```python
from build123d import *

# Parameters (mm, degrees)
F2_W      = 42.5
F2_H      = 40.5
F2_R      = 7.5
F8_DEPTH  = 2
F6_W      = 23.5
F6_H      = 40.5
F9_DEPTH  = 2
F5_W      = 23.5
F5_H      = 40.5
F10_DEPTH = 2
F0_W      = 42.5
F0_H      = 20.5
F11_DEPTH = 2
F7_W      = 1
F7_H      = 2
F12_DEPTH = 38.5
F13_DEPTH = 40.5
F14_R     = 0.99999


# Not quite as in the source:
# - a fillet or chamfer that OpenCascade refuses, or shapes differently, is made with other operations: its cross-section is extruded or revolved along the edge and cut away or added
# - a fillet or chamfer is up to 0.001 mm smaller than in the source, because OpenCascade refuses the exact size


with BuildPart() as f8:
    # F2 (on line) → F8 (new body)
    with BuildSketch(Plane.XZ.offset(10.25)):
        with Locations((0, 20.25)):
            Rectangle(F2_W, F2_H)
        with Locations((0, 20.25)):
            Circle(F2_R, mode=Mode.SUBTRACT)
    extrude(amount=-F8_DEPTH)

    # F6 (on line) → F9 (join)
    with BuildSketch(Plane(origin=(-21.25, 0, 0), x_dir=(0, -1, 0), z_dir=(-1, 0, 0))):
        with Locations((-1.5, 20.25)):
            Rectangle(F6_W, F6_H)
    extrude(amount=-F9_DEPTH)

    # F5 (on line) → F10 (join)
    with BuildSketch(Plane.YZ.offset(21.25)):
        with Locations((1.5, 20.25)):
            Rectangle(F5_W, F5_H)
    extrude(amount=-F10_DEPTH)

    # F0 (on Top) → F11 (join)
    with BuildSketch(Plane.XY):
        Rectangle(F0_W, F0_H)
    extrude(amount=F11_DEPTH)

    # F7 (on Top) → F12 (cut)
    with BuildSketch(Plane.XY):
        with Locations((-19.75, 11.25)):
            Rectangle(F7_W, F7_H)
        with Locations((19.75, 11.25)):
            Rectangle(F7_W, F7_H)
    extrude(amount=-F12_DEPTH, mode=Mode.SUBTRACT)

    # F7 (on Top) → F13 (cut)
    with BuildSketch(Plane.XY):
        with Locations((19.75, 11.25)):
            Rectangle(F7_W, F7_H)
        with Locations((-19.75, 11.25)):
            Rectangle(F7_W, F7_H)
    extrude(amount=F13_DEPTH, mode=Mode.SUBTRACT)

    # F14 (radius 1 in the source; OpenCascade refuses exactly that, so slightly less here)
    f14_edges = [f8.edges().sort_by_distance(p)[0] for p in [
        (0, -10.25, 0),
        (21.25, 1.5, 0),
        (21.25, 13.25, 20.25),
        (21.25, -10.25, 20.25),
        (-21.25, -10.25, 20.25),
        (-21.25, 1.5, 0),
    ]]
    fillet(f14_edges, radius=F14_R)

    # F15: fillet of radius 5.08 on 1 edges, made by hand

    # F15_s1 → F15_t2 (revolve, cut)
    with BuildSketch(Plane.XY.offset(20.25)):
        with BuildLine():
            ThreePointArc((11.5398019753, -10.25), (9.2859164414, -9.7226256161), (7.5, -8.25))
            Line((7.5, -8.25), (7.5, -10.25))
            Line((7.5, -10.25), (11.5398019753, -10.25))
        make_face()
    revolve(axis=Axis((0, -10.25, 20.25), (0, -1, 0)), mode=Mode.SUBTRACT)


solid = f8.part
```
For this review, take the finished solid that the model builds, in its own axes (mm). A direction names the side the tool comes from. Coordinates: 2 decimals unless noted, no trailing zeros. Order: outer loops, then holes, each group sorted by start corner. A loop starts at its lowest first (then second) coordinate and runs counter-clockwise, first axis right, second up. Notation, with made-up numbers: (-26, 10) -> (21, 10) arc R16 cw to (21, 23) -> close; hole circle Ø8 at (73.25, 0.5). An arc over 180 degrees is marked (long way). Answer as CSV lines item,"result".
Q1. Clearance check with flat-ended pins moving along their axes: pin 1 Ø1.5 at (x, y) = (-4, 5.5) entering from +Z; pin 2 Ø0.8 at (y, z) = (13, 21) entering from +X; pin 3 Ø19 at (x, z) = (7.5, 13) entering from +Y. State where each tip first meets the part, or that it passes through.
Model answer:
pin 1,"stops at z = 2"
pin 2,"stops at x = 21.19"
pin 3,"stops at y = -8.25"
Q2. We need section B-B (z = 3). State the section outline as (x, y) points.
Model answer:
outline,"(-21.25, -9.25) arc R1 ccw to (-20.25, -10.25) -> (20.25, -10.25) arc R1 ccw to (21.25, -9.25) -> (21.25, 12.25) arc R1 ccw to (20.25, 13.25) -> (19.25, 13.25) -> (19.25, 12.25) -> (20.25, 12.25) -> (20.25, 10.25) -> (19.25, 10.25) -> (19.25, -8.25) -> (-19.25, -8.25) -> (-19.25, 10.25) -> (-20.25, 10.25) -> (-20.25, 12.25) -> (-19.25, 12.25) -> (-19.25, 13.25) -> (-21.25, 13.25) -> close"
Q3. Wall thickness on line 1 along X through (y, z) = (-0.75, 33.5); line 2 along Y through (x, z) = (9, 35); line 3 along Z through (x, y) = (-6, -4.5): over which ranges is each line inside the solid? List them lowest first. Write a range as [from, to].
Model answer:
line 1,"x = [-21.25, -19.25], [19.25, 21.25]"
line 2,"y = [-10.25, -8.25]"
line 3,"z = [0, 2]"
Q4. For faces 1 (the face through (20, 12.25, 20)), 2 (the face through (0, -8.25, 30)), 3 (the face through (19.25, 13, 21)), list the 3-axis set-ups (+Z, -Z, +X, -X, +Y, -Y) from which the entire face can be reached by the end or side of a thin tool; tool diameter is ignored.
Model answer:
face 1,"+Z, -Z"
face 2,"+Z, +Y"
face 3,"+Z, -Z, +Y"
Q5. We need section A-A (y = -3). State the section outline as (x, z) points.
Model answer:
outline,"(-21.25, 1) arc R1 ccw to (-20.25, 0) -> (20.25, 0) arc R1 ccw to (21.25, 1) -> (21.25, 40.5) -> (19.25, 40.5) -> (19.25, 2) -> (-19.25, 2) -> (-19.25, 40.5) -> (-21.25, 40.5) -> close"
Q6. Draft analysis for pull direction X (two halves, no side actions). For faces 4 (the face through (20, 13.25, 20)), 5 (the face through (-19.25, 1, 22)), 6 (the face through (21.25, 1, 20)), state which applies: released by +X, released by -X, zero draft, split by the parting line, or undercut.
Model answer:
face 4,"zero draft"
face 5,"undercut"
face 6,"released by +X"
